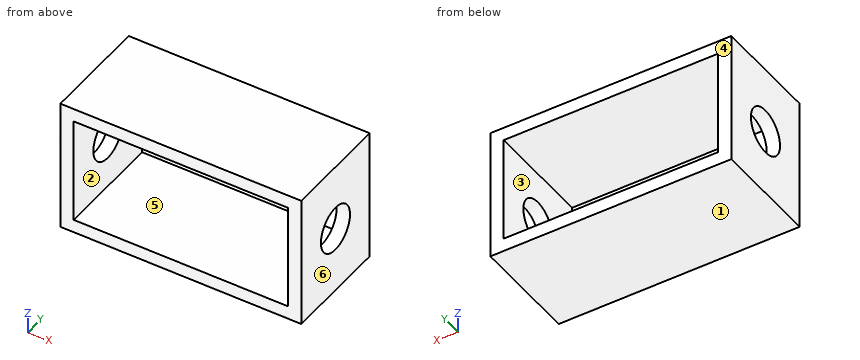
```python
from build123d import *

# Parameters (mm, degrees)
SKETCH1_W           = 45
SKETCH1_H           = 25
SKETCH1_W_2         = 40
SKETCH1_H_2         = 20
BOSS_EXTRUDE1_DEPTH = 2.5
SKETCH2_W           = 45
SKETCH2_H           = 25
SKETCH2_W_2         = 40
SKETCH2_H_2         = 20
BOSS_EXTRUDE2_DEPTH = 17.5
SKETCH3_R           = 4.25
CUT_EXTRUDE1_DEPTH  = 46


with BuildPart() as part:
    # Sketch1 → Boss-Extrude1 (new body)
    with BuildSketch(Plane(origin=(0, 0, 0), x_dir=(1, 0, 0), z_dir=(0, 1, 0))):
        Rectangle(SKETCH1_W, SKETCH1_H)
        Rectangle(SKETCH1_W_2, SKETCH1_H_2, mode=Mode.SUBTRACT)
    extrude(amount=BOSS_EXTRUDE1_DEPTH)

    # Sketch2 → Boss-Extrude2 (add)
    with BuildSketch(Plane(origin=(0, 2.5, 0), x_dir=(1, 0, 0), z_dir=(0, 1, 0))):
        Rectangle(SKETCH2_W, SKETCH2_H)
        Rectangle(SKETCH2_W_2, SKETCH2_H_2, mode=Mode.SUBTRACT)
    extrude(amount=BOSS_EXTRUDE2_DEPTH)

    # Sketch3 → Cut-Extrude1 (cut, through all)
    with BuildSketch(Plane(origin=(22.5, 0, 0), x_dir=(0, 0, -1), z_dir=(1, 0, 0))):
        with Locations((0, 10)):
            Circle(SKETCH3_R)
    extrude(amount=-CUT_EXTRUDE1_DEPTH, mode=Mode.SUBTRACT)


solid = part.part
```
Design review of the part built by this model. Coordinates are the model's own, in mm. Face numbers are marked on the shaded views. A direction names the side the tool comes from. Give positions to 0.01 mm unless a question says otherwise; leave off trailing zeros. Write each loop counter-clockwise with the first axis right and the second up, starting at its lowest first coordinate (ties: lowest second). Pieces come first, ordered by that corner, then holes.
(1) Clearance check with a flat-ended pin moving along its axis: pin 1 Ø7.5 at (y, z) = (10, 0) entering from +X. State where the tip first meets the part, or that it passes through.
Checked values:
pin 1: passes through
(2) Mouldability with a two-part tool opening along Z and no side actions: class the marked faces 1, 2, 3 and 4 as +Z half, -Z half, draft (parallel to the pull), parting line (faces both ways), or undercut.
Checked values:
face 1: -Z half
face 2: undercut
face 3: undercut
face 4: draft
(3) Tool access review of the marked faces 5 and 6: name each direction out of +Z, -Z, +X, -X, +Y, -Y from which nothing blocks a thin tool from reaching the whole face with its end or side.
Checked values:
face 5: +Y, -Y
face 6: +Z, -Z, +X, +Y, -Y
(4) Add section A-A (y = 10). Give the boundary of the cut face in (x, z).
Checked values:
outline: (-22.5, -12.5) - (22.5, -12.5) - (22.5, -4.25) - (20, -4.25) - (20, -10) - (-20, -10) - (-20, -4.25) - (-22.5, -4.25) - close; (-22.5, 4.25) - (-20, 4.25) - (-20, 10) - (20, 10) - (20, 4.25) - (22.5, 4.25) - (22.5, 12.5) - (-22.5, 12.5) - close
(5) Add section B-B (x = -3.5). Give the boundary of the cut face in (y, z), and give its area (3 significant figures).
Checked values:
outline: (0, -12.5) - (20, -12.5) - (20, -10) - (0, -10) - close; (0, 10) - (20, 10) - (20, 12.5) - (0, 12.5) - close
area: 100 mm2
(6) Add section C-C (z = 0). Give the boundary of the cut face in (x, y).
Checked values:
outline: (-22.5, 0) - (-20, 0) - (-20, 5.75) - (-22.5, 5.75) - close; (-22.5, 14.25) - (-20, 14.25) - (-20, 20) - (-22.5, 20) - close; (20, 0) - (22.5, 0) - (22.5, 5.75) - (20, 5.75) - close; (20, 14.25) - (22.5, 14.25) - (22.5, 20) - (20, 20) - close
(7) Add section D-D (y = 18.5). Give the boundary of the cut face in (x, z), and give its area (3 significant figures).
Checked values:
outline: (-22.5, -12.5) - (22.5, -12.5) - (22.5, 12.5) - (-22.5, 12.5) - close; hole (-20, -10) - (20, -10) - (20, 10) - (-20, 10) - close
area: 325 mm2
(8) Wall thickness on line 1 along X through (y, z) = (11.25, 6.5); line 2 along Z through (x, y) = (10.5, 18); line 3 along Y through (x, z) = (21.3, 0): over which ranges is each line inside the solid? List them lowest first.
Checked values:
line 1: x = -22.5 to -20, 20 to 22.5
line 2: z = -12.5 to -10, 10 to 12.5
line 3: y = 0 to 5.75, 14.25 to 20
